Can you work these out from the model? Positions are in its coordinate system, mm. Face numbers are marked on the shaded views. A direction names the side the tool comes from. Coordinates: 2 decimals unless noted, no trailing zeros. Loops run counter-clockwise (first coordinate to the right, second up) from the corner with the lowest first, then second, coordinate; pieces in that order, holes last. Notation, with made-up numbers: (45.25, 30.25) -> (73.25, 30.25) arc R23 ccw to (73.25, 69.25) -> close; hole circle Ø8 at (76, -14). An arc over 180 degrees is marked (long way). Use one line per item in the form item = value. Start each with the question number.
(1) On a 3-axis mill with a long thin cutter (end or side, diameter ignored), from which of +Z, -Z, +X, -X, +Y, -Y can I reach the whole of each face in a straight line? I mean the marked faces 1, 2, 3, 4 and 5. Say none if no direction works.
(2) Thinking about a two-plate mould opening in X: for the marked faces 6, 7 and 8, which applies, released by +X, released by -X, zero draft, split by the parting line, or undercut?
(3) Imagine slicing it at D-D (y = 8.5). List the corners of the cut face in (x, z) for me, plus the area to 3 significant figures.
(4) Imagine slicing it at B-B (z = -0.1). List the corners of the cut face in (x, y) for me, plus the area to 3 significant figures.
(5) Imagine slicing it at C-C (x = 0). List the corners of the cut face in (y, z) for me.
(6) Imagine slicing it at A-A (y = -1). List the corners of the cut face in (x, z) for me.
(7) I'm going to push flat-ended pins straight in: pin 1 (0.5 mm diameter, centred on x = -2, y = -1, fed in from -Z); pin 2 (1.9 mm diameter, centred on y = 6.5, z = 0, fed in from +X); pin 3 (0.6 mm diameter, centred on y = 9, z = -0.5, fed in from +X). Where does each tip first touch, or does it pass through?
(8) I need wall thicknesses on line 1 (Z direction, x = -0.9, y = 6.75); line 2 (Z direction, x = 0.9, y = 9); line 3 (Y direction, x = -1.6, z = 1.5). Which ranges of each line are inside material? Lowest first, please. Write a range as [from, to].
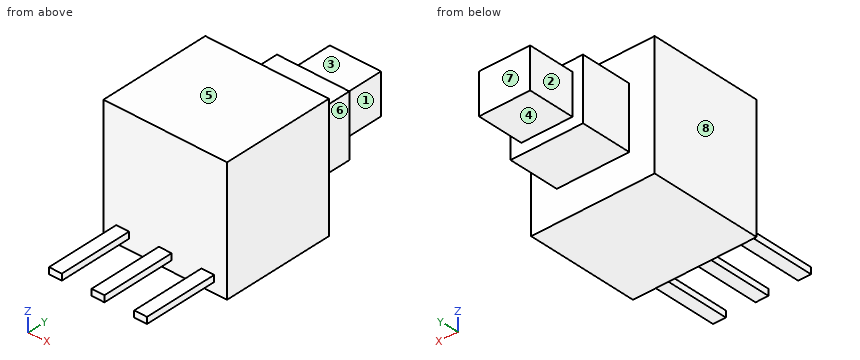
```python
from build123d import *

# Parameters (mm, degrees)
ESQUISSE1_W        = 5.8
ESQUISSE1_H        = 5.8
BOSS_EXTRU_1_DEPTH = 5.3
ESQUISSE2_W        = 3.4
ESQUISSE2_H        = 2.9
BOSS_EXTRU_2_DEPTH = 2.4
ESQUISSE4_W        = 2.4
ESQUISSE4_H        = 1.9
BOSS_EXTRU_3_DEPTH = 2.2
ESQUISSE5_W        = 0.6
ESQUISSE5_H        = 0.3
BOSS_EXTRU_4_DEPTH = 3.5


with BuildPart() as part:
    # Esquisse1 → Boss.-Extru.1 (new body)
    with BuildSketch(Plane(origin=(0, 0, 0), x_dir=(1, 0, 0), z_dir=(0, 1, 0))):
        Rectangle(ESQUISSE1_W, ESQUISSE1_H)
    extrude(amount=BOSS_EXTRU_1_DEPTH)

    # Esquisse2 → Boss.-Extru.2 (add)
    with BuildSketch(Plane(origin=(0, 5.3, 0), x_dir=(1, 0, 0), z_dir=(0, 1, 0))):
        Rectangle(ESQUISSE2_W, ESQUISSE2_H)
    extrude(amount=BOSS_EXTRU_2_DEPTH)

    # Esquisse4 → Boss.-Extru.3 (add)
    with BuildSketch(Plane(origin=(0, 7.7, 0), x_dir=(1, 0, 0), z_dir=(0, 1, 0))):
        Rectangle(ESQUISSE4_W, ESQUISSE4_H)
    extrude(amount=BOSS_EXTRU_3_DEPTH)

    # Esquisse5 → Boss.-Extru.4 (add)
    with BuildSketch(Plane.XZ):
        with Locations((0, -2.271834071)):
            Rectangle(ESQUISSE5_W, ESQUISSE5_H)
        with Locations((-2, -2.271834071)):
            Rectangle(ESQUISSE5_W, ESQUISSE5_H)
        with Locations((2, -2.271834071)):
            Rectangle(ESQUISSE5_W, ESQUISSE5_H)
    extrude(amount=BOSS_EXTRU_4_DEPTH)


solid = part.part
```
Worked out:
q1.face_1 = +Z, -Z, +X, +Y
q1.face_2 = +Z, -Z, -X, +Y
q1.face_3 = +Z, +X, -X, +Y
q1.face_4 = -Z, +X, -X, +Y
q1.face_5 = +Z, +X, -X, +Y, -Y
q2.face_6 = released by +X
q2.face_7 = zero draft
q2.face_8 = released by -X
q3.outline = (-1.2, -0.95) -> (1.2, -0.95) -> (1.2, 0.95) -> (-1.2, 0.95) -> close
q3.area = 4.56 mm2
q4.outline = (-2.9, 0) -> (2.9, 0) -> (2.9, 5.3) -> (1.7, 5.3) -> (1.7, 7.7) -> (1.2, 7.7) -> (1.2, 9.9) -> (-1.2, 9.9) -> (-1.2, 7.7) -> (-1.7, 7.7) -> (-1.7, 5.3) -> (-2.9, 5.3) -> close
q4.area = 44.2 mm2
q5.outline = (-3.5, -2.42) -> (0, -2.42) -> (0, -2.9) -> (5.3, -2.9) -> (5.3, -1.45) -> (7.7, -1.45) -> (7.7, -0.95) -> (9.9, -0.95) -> (9.9, 0.95) -> (7.7, 0.95) -> (7.7, 1.45) -> (5.3, 1.45) -> (5.3, 2.9) -> (0, 2.9) -> (0, -2.12) -> (-3.5, -2.12) -> close
q6.outline = (-2.3, -2.42) -> (-1.7, -2.42) -> (-1.7, -2.12) -> (-2.3, -2.12) -> close; (-0.3, -2.42) -> (0.3, -2.42) -> (0.3, -2.12) -> (-0.3, -2.12) -> close; (1.7, -2.42) -> (2.3, -2.42) -> (2.3, -2.12) -> (1.7, -2.12) -> close
q7.pin_1 = -2.42
q7.pin_2 = 1.7
q7.pin_3 = 1.2
q8.line_1 = [-1.45, 1.45]
q8.line_2 = [-0.95, 0.95]
q8.line_3 = [0, 5.3]
